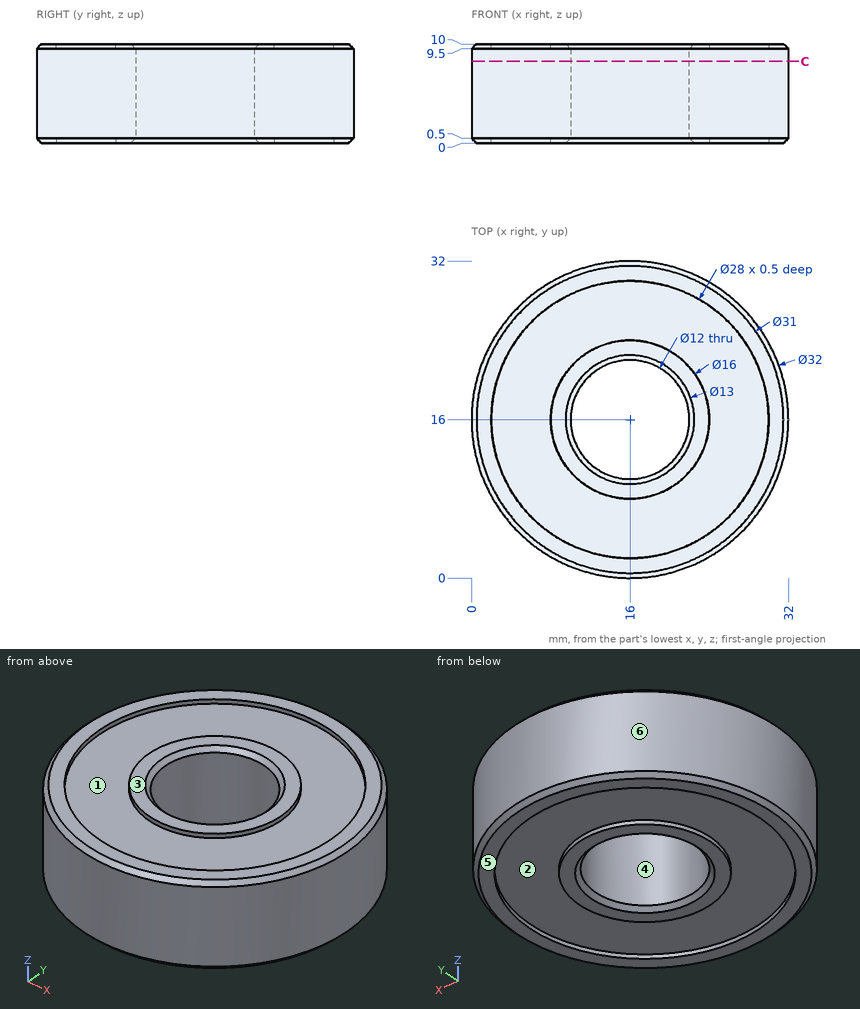
Answer from the drawing. Dimensions are ordinates in mm from the lowest x, y and z of the part. A direction names the side the tool comes from. Give positions to 0.01 mm unless a question says otherwise; leave off trailing zeros. Order: outer loops, then holes, each group sorted by start corner. A loop starts at its lowest first (then second) coordinate and runs counter-clockwise, first axis right, second up. Notation, with made-up numbers: (-29, 37.5) - (-4, 37.5) arc R17 cw to (-4, 66.5) - close; hole circle Ø10 at (-27.75, 68.25). An arc over 180 degrees is marked (long way). One line per item, written item: value. Start each with the question number.
1. Which of the six approach directions +Z, -Z, +X, -X, +Y, -Y give full straight-line access (tool end or side, diameter ignored) to the marked faces 1, 2 and 3?
2. For a pull along Y with two mould halves and no side action, classify the marked faces 4, 5 and 6 as released by +Y, released by -Y, zero draft, split by the parting line, or undercut.
3. Consider line 1 (Y direction, x = 16, z = 9.7); line 2 (Y direction, x = 16, z = 4); line 3 (Y direction, x = 16, z = 9.8). Determine where each line is inside the solid, lowest interval first.
4. Each of these flat-tipped pins is pushed along its axis until it touches: pin 1 Ø6 at (y, z) = (26.5, 9) entering from -X; pin 2 Ø3 at (y, z) = (7, 4.5) entering from +X; pin 3 Ø6 at (x, z) = (12.5, 8) entering from +Y. Where does it stop, or does it pass through?
5. Section C-C, the plane z = 8.25 is taken. Write down the section's boundary in (x, y).
Filled sheet:
1. face 1: +Z
1. face 2: -Z
1. face 3: +Z, +X, -X, +Y, -Y
2. face 4: undercut
2. face 5: zero draft
2. face 6: split by the parting line
3. line 1: 0.2 to 2, 8 to 9.8, 22.2 to 24, 30 to 31.8
3. line 2: 0 to 10, 22 to 32
3. line 3: 0.3 to 2, 8 to 9.7, 22.3 to 24, 30 to 31.7
4. pin 1: x = 1.87
4. pin 2: x = 30.13
4. pin 3: y = 31.99
5. outline: circle Ø32 at (16, 16); hole circle Ø12 at (16, 16)
